from build123d import *


with BuildPart() as part:
    # Sketch2 → Revolve1 (revolve)
    with BuildSketch(Plane.XY):
        with BuildLine():
            Line((2, 2.5), (2, -2.5))
            Line((2, -2.5), (6, -2.5))
            Line((6, -2.5), (6, -2.3))
            ThreePointArc((6, -2.3), (4.935246844, -1.414604424), (4.5, -0.1))
            Line((4.5, -0.1), (4.5, 0.1))
            ThreePointArc((4.5, 0.1), (4.935246844, 1.414604424), (6, 2.3))
            Line((6, 2.3), (6, 2.5))
            Line((6, 2.5), (2, 2.5))
        make_face()
    revolve(axis=Axis((0, -2.5, 0), (0, 1, 0)))


solid = part.part
For this review, take the finished solid that the model builds, in its own axes (mm). Coordinates: 2 decimals unless noted, no trailing zeros. Loops run counter-clockwise (first coordinate to the right, second up) from the corner with the lowest first, then second, coordinate; pieces in that order, holes last. Notation, with made-up numbers: (19.25, -25) - (59.25, -25) arc R14 ccw to (59.25, -8) - close; hole circle Ø5 at (79, 50). An arc over 180 degrees is marked (long way). Return JSON: item names as keys, results as strings.
Item 1: Take a section at D-D (y = -0.35). Give the boundary of the cut face in (x, z), then the cut area to 3 significant figures.
Determined:
{"outline": "circle Ø9.05 at (0, 0); hole circle Ø4 at (0, 0)", "area": "51.7 mm2"}
Item 2: Mouldability with a two-part tool opening along Z and no side actions: class faces 1 (the cylindrical face through (0, 0, 2)), 2 (the flat face through (-3, -2.5, 0)) as pulls with the +Z half, pulls with the -Z half, needs draft (parallel to the pull), parting line crosses it, or undercut.
Determined:
{"face 1": "undercut", "face 2": "needs draft"}
Item 3: Take a section at A-A (x = 0). Give the boundary of the cut face in (y, z).
Determined:
{"outline": "(-2.5, -6) - (-2.3, -6) arc R2.52 cw to (-0.1, -4.5) - (0.1, -4.5) arc R2.52 cw to (2.3, -6) - (2.5, -6) - (2.5, -2) - (-2.5, -2) - close; (-2.5, 2) - (2.5, 2) - (2.5, 6) - (2.3, 6) arc R2.52 cw to (0.1, 4.5) - (-0.1, 4.5) arc R2.52 cw to (-2.3, 6) - (-2.5, 6) - close"}
Item 4: Take a section at B-B (z = 0). Give the boundary of the cut face in (x, y), then the cut area to 3 significant figures.
Determined:
{"outline": "(-6, -2.5) - (-2, -2.5) - (-2, 2.5) - (-6, 2.5) - (-6, 2.3) arc R2.52 cw to (-4.5, 0.1) - (-4.5, -0.1) arc R2.52 cw to (-6, -2.3) - close; (2, -2.5) - (6, -2.5) - (6, -2.3) arc R2.52 cw to (4.5, -0.1) - (4.5, 0.1) arc R2.52 cw to (6, 2.3) - (6, 2.5) - (2, 2.5) - close", "area": "30.1 mm2"}
Item 5: Take a section at C-C (y = -1.25). Give the boundary of the cut face in (x, z), then the cut area to 3 significant figures.
Determined:
{"outline": "circle Ø9.66 at (0, 0); hole circle Ø4 at (0, 0)", "area": "60.8 mm2"}
Item 6: For line 1 (X direction, y = -1.2, z = 0); line 2 (X direction, y = 0.3, z = -1.75); line 3 (Z direction, x = 0, y = -0.95), list the stretches that pass through material, from the lowest coordinate up.
Determined:
{"line 1": "x = -4.8 to -2, 2 to 4.8", "line 2": "x = -4.16 to -0.97, 0.97 to 4.16", "line 3": "z = -4.69 to -2, 2 to 4.69"}
Item 7: Insertion check: pin 1 (4.5 mm diameter, centred on x = 0, z = 0, fed in from -Y); pin 2 (3 mm diameter, centred on x = 1, y = 1, fed in from -Z); pin 3 (3 mm diameter, centred on x = -3, y = 2, fed in from +Z). Each pin has a flat end and moves straight along its axis. Give the tip position at first contact, or say it passes through.
Determined:
{"pin 1": "stops at y = -2.5", "pin 2": "stops at z = -5.99", "pin 3": "stops at z = 5.8"}
